Could you check a few things on this model? Use its own coordinates, in mm. A direction names the side the tool comes from. Coordinates: 2 decimals unless noted, no trailing zeros. Loops run counter-clockwise (first coordinate to the right, second up) from the corner with the lowest first, then second, coordinate; pieces in that order, holes last. Notation, with made-up numbers: (54.25, 1.5) -> (60.25, 1.5) arc R17 cw to (60.25, 7.5) -> close; hole circle Ø10 at (-14, 23.25). An arc over 180 degrees is marked (long way). One line per question, with ' | ' between items.
```python
from build123d import *

# Parameters (mm, degrees)
SKETCH1_W           = 25.4
SKETCH1_H           = 25.4
SKETCH1_W_2         = 22.225
SKETCH1_H_2         = 22.225
BOSS_EXTRUDE1_DEPTH = 152.4
SKETCH2_R           = 6.35
CUT_EXTRUDE1_DEPTH  = 127
SKETCH3_R           = 6.35
CUT_EXTRUDE2_DEPTH  = 127
SKETCH4_R           = 6.35
CUT_EXTRUDE3_DEPTH  = 127
SKETCH5_R           = 6.35
CUT_EXTRUDE4_DEPTH  = 127


with BuildPart() as part:
    # Sketch1 → Boss-Extrude1 (new body)
    with BuildSketch(Plane(origin=(0, 0, 0), x_dir=(1, 0, 0), z_dir=(0, 1, 0))):
        Rectangle(SKETCH1_W, SKETCH1_H)
        Rectangle(SKETCH1_W_2, SKETCH1_H_2, mode=Mode.SUBTRACT)
    extrude(amount=BOSS_EXTRUDE1_DEPTH)

    # Sketch2 → Cut-Extrude1 (cut)
    with BuildSketch(Plane(origin=(0, 0, -12.7), x_dir=(-1, 0, 0), z_dir=(0, 0, -1))):
        with Locations((0, 139.7)):
            Circle(SKETCH2_R)
    extrude(amount=-CUT_EXTRUDE1_DEPTH, mode=Mode.SUBTRACT)

    # Sketch3 → Cut-Extrude2 (cut)
    with BuildSketch(Plane(origin=(12.7, 0, 0), x_dir=(0, 0, -1), z_dir=(1, 0, 0))):
        with Locations((0, 127)):
            Circle(SKETCH3_R)
    extrude(amount=-CUT_EXTRUDE2_DEPTH, mode=Mode.SUBTRACT)

    # Sketch4 → Cut-Extrude3 (cut)
    with BuildSketch(Plane(origin=(0, 0, -12.7), x_dir=(-1, 0, 0), z_dir=(0, 0, -1))):
        with Locations((0, 12.7)):
            Circle(SKETCH4_R)
    extrude(amount=-CUT_EXTRUDE3_DEPTH, mode=Mode.SUBTRACT)

    # Sketch5 → Cut-Extrude4 (cut)
    with BuildSketch(Plane(origin=(12.7, 0, 0), x_dir=(0, 0, -1), z_dir=(1, 0, 0))):
        with Locations((0, 25.4)):
            Circle(SKETCH5_R)
    extrude(amount=-CUT_EXTRUDE4_DEPTH, mode=Mode.SUBTRACT)


solid = part.part
```
Q1. Please list where these lines run through material, in increasing order: L1, parallel to Y at x = 12.2, z = 0; L2, parallel to X at y = 21.5, z = 11. Write a range as [from, to].
Values follow:
L1: y = [0, 19.05], [31.75, 120.65], [133.35, 152.4] | L2: x = [-12.7, -11.11], [11.11, 12.7]
Q2. For pin 1 (14.5 mm diameter, centred on y = 127, z = 0, fed in from +X), with a flat end and sliding along its axis, tell me the tip position at first contact or that it passes through.
Values follow:
pin 1: stops at x = 12.7
Q3. Imagine slicing it at C-C on z = 0. Write out the boundary of the cut face in (x, y), plus the area to 3 significant figures.
Values follow:
outline: (-12.7, 0) -> (-11.11, 0) -> (-11.11, 19.05) -> (-12.7, 19.05) -> close; (-12.7, 31.75) -> (-11.11, 31.75) -> (-11.11, 120.65) -> (-12.7, 120.65) -> close; (-12.7, 133.35) -> (-11.11, 133.35) -> (-11.11, 152.4) -> (-12.7, 152.4) -> close; (11.11, 0) -> (12.7, 0) -> (12.7, 19.05) -> (11.11, 19.05) -> close; (11.11, 31.75) -> (12.7, 31.75) -> (12.7, 120.65) -> (11.11, 120.65) -> close; (11.11, 133.35) -> (12.7, 133.35) -> (12.7, 152.4) -> (11.11, 152.4) -> close | area: 403 mm2
Q4. We'd pull the mould along Y, two halves only. Please class faces 1 (the face through (-3.414, 18.054, -11.917)), 2 (the face through (-11.3, 152.4, -0.1)), 3 (the face through (12.7, 75, 0)): released by +Y, released by -Y, zero draft, split by the parting line, or undercut.
Values follow:
face 1: undercut | face 2: released by +Y | face 3: zero draft
Q5. Imagine slicing it at B-B on y = 25.4. Write out the boundary of the cut face in (x, z), plus the area to 3 significant figures.
Values follow:
outline: (-12.7, -12.7) -> (12.7, -12.7) -> (12.7, -6.35) -> (11.11, -6.35) -> (11.11, -11.11) -> (-11.11, -11.11) -> (-11.11, -6.35) -> (-12.7, -6.35) -> close; (-12.7, 6.35) -> (-11.11, 6.35) -> (-11.11, 11.11) -> (11.11, 11.11) -> (11.11, 6.35) -> (12.7, 6.35) -> (12.7, 12.7) -> (-12.7, 12.7) -> close | area: 111 mm2
Q6. For faces 4 (the face through (11.112, 75, 0)), 5 (the face through (1.38, 133.5, 11.9)), which set-ups out of +Z, -Z, +X, -X, +Y, -Y let a thin tool reach every point of the face, with its end or its side?
Values follow:
face 4: +Y, -Y | face 5: +Z, -Z
Q7. Imagine slicing it at D-D on y = 77. Write out the boundary of the cut face in (x, z), plus the area to 3 significant figures.
Values follow:
outline: (-12.7, -12.7) -> (12.7, -12.7) -> (12.7, 12.7) -> (-12.7, 12.7) -> close; hole (-11.11, -11.11) -> (11.11, -11.11) -> (11.11, 11.11) -> (-11.11, 11.11) -> close | area: 151 mm2
Q8. Imagine slicing it at A-A on z = -8.25. Write out the boundary of the cut face in (x, y).
Values follow:
outline: (-12.7, 0) -> (-11.11, 0) -> (-11.11, 152.4) -> (-12.7, 152.4) -> close; (11.11, 0) -> (12.7, 0) -> (12.7, 152.4) -> (11.11, 152.4) -> close
